from build123d import *

# Parameters (mm, degrees)
SKETCH_1_W          = 60
SKETCH_1_H          = 45
EXTRUDE_1_DEPTH     = 80
FILLET_1_R          = 8
SKETCH_2_W          = 15
SKETCH_2_H          = 15
CUT_EXTRUDE_1_DEPTH = 110.658560997
SKETCH_3_R          = 2.5
CUT_EXTRUDE_2_DEPTH = 5
EXTRUDE_2_DEPTH     = 12


with BuildPart() as part:
    # ｽｹｯﾁ1 → 押し出し1 (new body)
    with BuildSketch(Plane.XY):
        with Locations((30, 22.5)):
            Rectangle(SKETCH_1_W, SKETCH_1_H)
    extrude(amount=EXTRUDE_1_DEPTH)

    # ﾌｨﾚｯﾄ1
    fillet_1_edges = [part.edges().sort_by_distance(p)[0] for p in [
        (60, 22.5, 80),
        (0, 22.5, 80),
        (60, 22.5, 0),
        (0, 22.5, 0),
    ]]
    fillet(fillet_1_edges, radius=FILLET_1_R)

    # ｽｹｯﾁ2 → ｶｯﾄ - 押し出し1 (cut, through all)
    with BuildSketch(Plane.XY.offset(80)):
        with Locations((52.5, 7.5)):
            Rectangle(SKETCH_2_W, SKETCH_2_H)
        with Locations((7.5, 7.5)):
            Rectangle(SKETCH_2_W, SKETCH_2_H)
    extrude(amount=-CUT_EXTRUDE_1_DEPTH, mode=Mode.SUBTRACT)

    # ｽｹｯﾁ3 → ｶｯﾄ - 押し出し2 (cut)
    with BuildSketch(Plane.XZ):
        with Locations(Location((41.136931804, 51.136931804, 0), (0, 0, 270))):
            Circle(SKETCH_3_R)
        with Locations(Location((41.136931804, 28.863068196, 0), (0, 0, 270))):
            Circle(SKETCH_3_R)
        with Locations(Location((18.863068196, 51.136931804, 0), (0, 0, 270))):
            Circle(SKETCH_3_R)
        with Locations(Location((18.863068196, 28.863068196, 0), (0, 0, 270))):
            Circle(SKETCH_3_R)
    extrude(amount=-CUT_EXTRUDE_2_DEPTH, mode=Mode.SUBTRACT)

    # ｽｹｯﾁ4 → 押し出し2 (add)
    with BuildSketch(Plane(origin=(0, 45, 0), x_dir=(-1, 0, 0), z_dir=(0, 1, 0))):
        Polygon((-50, 29), (-20, 29), (-20, 37), (-42, 37), (-42, 57), (-50, 57), align=None)
        Polygon((-10, 23), (-10, 51), (-40, 51), (-40, 43), (-18, 43), (-18, 23), align=None)
    extrude(amount=EXTRUDE_2_DEPTH)


solid = part.part
Read the model definition and answer for the solid it produces. Units are mm, in the model's axes. A direction names the side the tool comes from. Coordinates: 2 decimals unless noted, no trailing zeros. Loops run counter-clockwise (first coordinate to the right, second up) from the corner with the lowest first, then second, coordinate; pieces in that order, holes last. Notation, with made-up numbers: (17.5, 66.5) -> (75.5, 66.5) arc R31 ccw to (75.5, 97.5) -> close; hole circle Ø11 at (72, 65). An arc over 180 degrees is marked (long way). Write item = value, one per line. Start each with the question number.
1) The mould has two halves that part along X. Classify faces 5 (the face through (50, 51, 43)), 6 (the face through (40, 51, 47)), 7 (the face through (42, 51, 47)), 8 (the face through (30, 23, 0)): pulls with the +X half, pulls with the -X half, needs draft (parallel to the pull), parting line crosses it, or undercut.
2) For faces 1 (the face through (31, 51, 37)), 2 (the face through (14, 51, 23)), 3 (the face through (18, 51, 33)), 4 (the face through (18.973, 2.465, 53.635)), determine the directions among +Z, -Z, +X, -X, +Y, -Y from which every point of the face is accessible in a straight line to the end or side of a thin tool.
3) The part is cut by section D-D, the plane z = 19.5. Determine the outline of the cut face in (x, y), plus the area to 3 significant figures.
4) The part is cut by section C-C, the plane x = 31. Determine the outline of the cut face in (y, z), plus the area to 3 significant figures.
5) The part is cut by section B-B, the plane z = 44. Determine the outline of the cut face in (x, y).
6) The part is cut by section A-A, the plane y = 50. Determine the outline of the cut face in (x, z), plus the area to 3 significant figures.
7) Find the intervals of material crossed by L1, parallel to Y at x = 14, z = 28; L2, parallel to Y at x = 52, z = 8; L3, parallel to Z at x = 43, y = 45.5, in increasing order. Write a range as from..to.
8) Given P1, Ø8, axis at y = 9, z = 31.5, coming from the +X side; P2, Ø3.5, axis at x = 28.5, y = 54, coming from the +Z side; P3, Ø1.5, axis at x = 9.5, z = 60, coming from the -Y side, each flat-ended and moving along its own axis, determine where each tip first touches the part or whether it passes through.
Result:
q1.face_5 = pulls with the +X half
q1.face_6 = undercut
q1.face_7 = undercut
q1.face_8 = needs draft
q2.face_1 = +Y
q2.face_2 = -Z, +X, -X, +Y
q2.face_3 = -Z, +Y
q2.face_4 = -Y
q3.outline = (0, 15) -> (15, 15) -> (15, 0) -> (45, 0) -> (45, 15) -> (60, 15) -> (60, 45) -> (0, 45) -> close
q3.area = 2,250 mm²
q4.outline = (0, 0) -> (45, 0) -> (45, 29) -> (57, 29) -> (57, 37) -> (45, 37) -> (45, 43) -> (57, 43) -> (57, 51) -> (45, 51) -> (45, 80) -> (0, 80) -> close
q4.area = 3,790 mm²
q5.outline = (0, 15) -> (15, 15) -> (15, 0) -> (45, 0) -> (45, 15) -> (60, 15) -> (60, 45) -> (50, 45) -> (50, 57) -> (42, 57) -> (42, 45) -> (40, 45) -> (40, 57) -> (10, 57) -> (10, 45) -> (0, 45) -> close
q6.outline = (10, 23) -> (18, 23) -> (18, 43) -> (40, 43) -> (40, 51) -> (10, 51) -> close; (20, 29) -> (50, 29) -> (50, 57) -> (42, 57) -> (42, 37) -> (20, 37) -> close
q6.area = 800 mm²
q7.L1 = 15..57
q7.L2 = 15..45
q7.L3 = 29..57
q8.P1 = 45
q8.P2 = 51
q8.P3 = 15
